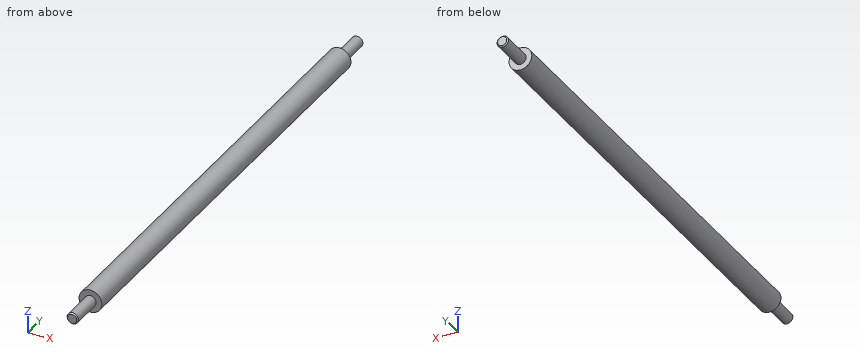
Autodesk Inventor part; units mm, degrees
ref_plane "YZ Plane" through (0, 0, 0) normal (1, 0, 0) x (0, 1, 0)
ref_plane "XZ Plane" through (0, 0, 0) normal (0, 1, 0) x (-1, 0, 0)
ref_plane "XY Plane" through (0, 0, 0) normal (0, 0, 1) x (1, 0, 0)
sketch "Boceto1" plane through (0, 0, 0) normal (0, 0, 1) x (1, 0, 0)
  line L0 (0, -70.5) -> (0, 70.5)
  line L1 (0, 70.5) -> (-1.5, 70.5)
  line L2 (-1.5, 70.5) -> (-1.5, 61.5)
  line L3 (-1.5, 61.5) -> (-3, 61.5)
  line L4 (-3, 61.5) -> (-3, -61.5)
  line L5 (-3, -61.5) -> (-1.5, -61.5)
  line L6 (-1.5, -61.5) -> (-1.5, -70.5)
  line L7 (-1.5, -70.5) -> (0, -70.5)
  point P0 (0, 0)
  point P1 (0, 0)
  dimension "d1" = 3
  dimension "d2" = 6
  dimension "d3" = 9
  dimension "d4" = 123
  dimension "d8" = 9
revolve "Revolución1" add sketch "Boceto1" angle 360 about axis through (0, -70.5, 0) along (0, 1, 0)
thread "Rosca1"
chamfer "Chaflán1" distance 0.3067 angle 45 2 edges at (1.5, 70.5, 0) (1.5, -70.5, 0)
properties part number "Columnas" material "Aluminum 7075"
Model file for the job. Use its own axes, mm. Round coordinates to 2 decimals unless told otherwise and drop trailing zeros. Loops run counter-clockwise (first coordinate to the right, second up) from the corner with the lowest first, then second, coordinate; pieces in that order, holes last.
1. Drop flat-ended pins along their axis: P1, Ø1.5, axis at x = 1.5, y = -9.5, coming from the -Z side; P2, Ø1, axis at x = -2, y = 44.5, coming from the -Z side; P3, Ø1, axis at y = -51.5, z = 1, coming from the -X side; P4, Ø3, axis at x = 1.5, z = -1.5, coming from the +Y side. Give the stop position or say it passes through.
Check values:
P1: stops at z = -2.9
P2: stops at z = -2.6
P3: stops at x = -2.96
P4: stops at y = 70.5
2. Band-saw the part on A-A, the plane x = 0. List the corners of the cut face in (y, z).
Check values:
outline: (-70.5, -1.19) - (-70.19, -1.5) - (-61.5, -1.5) - (-61.5, -3) - (61.5, -3) - (61.5, -1.5) - (70.19, -1.5) - (70.5, -1.19) - (70.5, 1.19) - (70.19, 1.5) - (61.5, 1.5) - (61.5, 3) - (-61.5, 3) - (-61.5, 1.5) - (-70.19, 1.5) - (-70.5, 1.19) - close
3. Band-saw the part on C-C, the plane y = 3. List the corners of the cut face in (x, z).
Check values:
outline: circle Ø6 at (0, 0)
4. Wall check: probe 1 along X at (y, z) = (-1, -0.2); probe 2 along Y at (x, z) = (1.75, -1.95); probe 3 along Z at (x, y) = (0, -64). Give the ranges that are in metal, low to high.
Check values:
probe 1: x = -2.99 to 2.99
probe 2: y = -61.5 to 61.5
probe 3: z = -1.5 to 1.5
5. Band-saw the part on B-B, the plane z = 0. List the corners of the cut face in (x, y).
Check values:
outline: (-3, -61.5) - (-1.5, -61.5) - (-1.5, -70.19) - (-1.19, -70.5) - (1.19, -70.5) - (1.5, -70.19) - (1.5, -61.5) - (3, -61.5) - (3, 61.5) - (1.5, 61.5) - (1.5, 70.19) - (1.19, 70.5) - (-1.19, 70.5) - (-1.5, 70.19) - (-1.5, 61.5) - (-3, 61.5) - close
